Autodesk Inventor part; units mm, degrees
ref_plane "YZ Plane" through (0, 0, 0) normal (1, 0, 0) x (0, 1, 0)
ref_plane "XZ Plane" through (0, 0, 0) normal (0, 1, 0) x (-1, 0, 0)
ref_plane "XY Plane" through (0, 0, 0) normal (0, 0, 1) x (1, 0, 0)
sketch "Эскиз1" plane through (0, 0, 0) normal (0, 0, 1) x (1, 0, 0)
  line L0 (0, 0) -> (110, 0)
  line L1 (0, 0) -> (15, 0)
  line L2 (15, 0) -> (-15, 0)
  line L3 (-15, 0) -> (-15, 1500)
  line L4 (-15, 1500) -> (15, 1500)
  line L5 (15, 1500) -> (15, 0)
  line L6 (110, 0) -> (95, 0)
  line L7 (95, 0) -> (125, 0)
  line L8 (125, 0) -> (125, 1500)
  line L9 (125, 1500) -> (95, 1500)
  line L10 (95, 1500) -> (95, 0)
  line L11 (0, 0) -> (-90, 0)
  line L12 (-90, 0) -> (-90, -30)
  line L13 (125, 0) -> (215, 0)
  line L14 (215, 0) -> (215, -30)
  line L15 (215, -30) -> (-90, -30)
  point P0 (-15, 0)
  dimension "d0" = 110
  dimension "d1" = 15
  dimension "d2" = 30
  dimension "d3" = 1500
  dimension "d4" = 15
  dimension "d5" = 30
  dimension "d6" = 1500
  dimension "d7" = 90
  dimension "d8" = 30
  dimension "d9" = 90
extrude "Выдавливание1" add sketch "Эскиз1" along normal blind 40
sketch "Эскиз2" plane through (-90, 0, 0) normal (0, 1, 0) x (1, 0, 0)
  line L0 (185, -40) -> (105, -40)
  line L1 (-191.3354, 280) -> (0, 0)
  line L2 (305, 0) -> (305, -40)
  line L3 (480.4002, 280) -> (305, 0)
  line L4 (445, 280) -> (269.5998, 0)
  line L5 (0, 0) -> (305, 0)
  line L6 (36.3354, 0) -> (-155, 280)
  line L7 (-191.3354, 280) -> (-155, 280)
  line L8 (445, 280) -> (480.4002, 280)
  line L9 (-155, 280) -> (445, 280)
  line L10 (0, 0) -> (0, -40)
  line L11 (0, 0) -> (36.3354, 0)
  line L12 (305, 0) -> (269.5998, 0)
  line L13 (305, 0) -> (215, 0)
  line L14 (185, 0) -> (105, 0)
  line L15 (145, 0) -> (145, 280)
  line L16 (270.8246, -0.1173) -> (29.7017, -0.1173)
  line L17 (-155, 280) -> (-179.7693, 263.0742)
  line L18 (445, 280) -> (470.4236, 264.0739)
  point P0 (90, 0)
  point P1 (269.5998, 0)
  dimension "d26" = 600
  dimension "d28" = 30
  dimension "d29" = 30
extrude "Выдавливание2" add sketch "Эскиз2" against normal blind 30 contours L17 L6 L5 L1 | L18 L3 L5 L4
sketch "Эскиз3" plane through (0, 0, 40) normal (0, 0, 1) x (1, 0, 0)
  line L0 (-15, 0) -> (-15, 400)
  line L1 (-15, 1500) -> (-15, 0)
  line L2 (-15, 400) -> (125, 400)
  line L3 (125, 0) -> (125, 1500)
  line L4 (125, 400) -> (125, 370)
  line L5 (125, 370) -> (-15, 370)
  point P0 (0, 0)
  point P1 (-15, 370)
  dimension "d22" = 400
  dimension "d23" = 30
extrude "Выдавливание3" add sketch "Эскиз3" against normal blind 80
properties part number "Стойка"
Part model, mm, in its own coordinate system. A direction names the side the tool comes from. Give positions to 0.01 mm unless a question says otherwise; leave off trailing zeros. Loops run counter-clockwise (first coordinate to the right, second up) from the corner with the lowest first, then second, coordinate; pieces in that order, holes last. Notation, with made-up numbers: (66, -34) -> (96, -34) arc R22 ccw to (96, 1) -> close; hole circle Ø1 at (76.25, -11.5). An arc over 180 degrees is marked (long way). Write each question's results on one line, items separated by ' | '. Start each with the question number.
Q1. Band-saw the part on B-B on z = -215. List the corners of the cut face in (x, y), plus the area to 3 significant figures.
Q2. Pull direction X, two halves, no side cores. Call faces 4 (the face through (268.53, -14.79, -141.96)), 5 (the face through (0, 958, 0)), 6 (the face through (298.87, -14.79, -133.885)): +X half, -X half, draft (parallel to the pull), parting line (faces both ways), or undercut.
Q3. Band-saw the part on A-A on y = 670.5. List the corners of the cut face in (x, z), plus the area to 3 significant figures.
Q4. Which spindle directions (+Z, -Z, +X, -X, +Y, -Y) get a long thin tool onto all of the face, cutting with end or side? Do faces 1 (the face through (-15, 740, 26)), 2 (the face through (-147.993, -14.79, -138.04)), 3 (the face through (54, 0, 20)). Say none if no direction does.
Q5. Wall check: L1, parallel to X at y = 1301.5, z = 27.5; L2, parallel to Y at x = 7, z = -29.5; L3, parallel to Y at x = -90.5, z = -39.5. Give the ranges that are in metal, low to high.
Q6. Band-saw the part on D-D on x = -74.5. List the corners of the cut face in (y, z), plus the area to 3 significant figures.
Q7. Band-saw the part on C-C on x = -198.5. List the corners of the cut face in (y, z), plus the area to 3 significant figures.
Q8. Pin check, flat tips, straight feed: P1, Ø24, axis at y = 763, z = 18, coming from the -X side; P2, Ø12, axis at x = 47.5, z = 16, coming from the +Y side; P3, Ø15, axis at y = -18.5, z = 26.5, coming from the -X side. Stop position of each tip, or through.
Results are:
1) outline: (-236.92, -30) -> (-200.58, -30) -> (-200.58, 0) -> (-236.92, 0) -> close; (314.28, -30) -> (349.68, -30) -> (349.68, 0) -> (314.28, 0) -> close | area: 2,150 mm²
2) face 4: undercut | face 5: draft | face 6: +X half
3) outline: (-15, 0) -> (15, 0) -> (15, 40) -> (-15, 40) -> close; (95, 0) -> (125, 0) -> (125, 40) -> (95, 40) -> close | area: 2,400 mm²
4) face 1: +Z, -Z, -X, +Y | face 2: -Z, +Y, -Y | face 3: +Z, -Z
5) L1: x = -15 to 15, 95 to 125 | L2: y = 370 to 400 | L3: y = -30 to 0
6) outline: (-30, -30.49) -> (0, -30.49) -> (0, 40) -> (-30, 40) -> close | area: 2,110 mm²
7) outline: (-30, -211.95) -> (0, -211.95) -> (0, -158.78) -> (-30, -158.78) -> close | area: 1,600 mm²
8) P1: stops at x = -15 | P2: stops at y = 400 | P3: stops at x = -90
